Autodesk Fusion 360 part; units mm, degrees
sketch "Sketch1" plane through (0, 0, 0) normal (0, 0, 1) x (1, 0, 0)
  line L0 (0, 0) -> (74, 0)
  line L1 (74, 0) -> (74, 83)
  line L2 (74, 83) -> (0, 83)
  line L3 (0, 83) -> (0, 0)
  dimension "d6" = 74
  dimension "d7" = 83
extrude "Extrude1" add sketch "Sketch1" along normal blind 5
sketch "Sketch2" plane through (0, 0, 0) normal (0, -1, 0) x (1, 0, 0)
  line L0 (0, 0) -> (74, 0)
  line L1 (74, 0) -> (74, 5)
  line L2 (74, 5) -> (0, 5)
  line L3 (0, 5) -> (0, 0)
  line L4 (0, 5) -> (6.7273, 5)
  line L5 (6.7273, 5) -> (6.7273, 0)
  line L6 (6.7273, 0) -> (0, 0)
  line L7 (0, 0) -> (0, 5)
  line L8 (20.1818, 0) -> (13.4545, 0)
  line L9 (13.4545, 0) -> (13.4545, 5)
  line L10 (20.1818, 5) -> (20.1818, 0)
  line L11 (13.4545, 5) -> (20.1818, 5)
  line L12 (33.6364, 0) -> (26.9091, 0)
  line L13 (26.9091, 0) -> (26.9091, 5)
  line L14 (33.6364, 5) -> (33.6364, 0)
  line L15 (26.9091, 5) -> (33.6364, 5)
  line L16 (47.0909, 0) -> (40.3636, 0)
  line L17 (40.3636, 0) -> (40.3636, 5)
  line L18 (47.0909, 5) -> (47.0909, 0)
  line L19 (40.3636, 5) -> (47.0909, 5)
  line L20 (60.5455, 0) -> (53.8182, 0)
  line L21 (53.8182, 0) -> (53.8182, 5)
  line L22 (60.5455, 5) -> (60.5455, 0)
  line L23 (53.8182, 5) -> (60.5455, 5)
  line L24 (74, 0) -> (67.2727, 0)
  line L25 (67.2727, 0) -> (67.2727, 5)
  line L26 (74, 5) -> (74, 0)
  line L27 (67.2727, 5) -> (74, 5)
  dimension "d10" = 6.7273
  dimension "d13" = 67.2727
  dimension "d14" = 0
extrude "Extrude2" add sketch "Sketch2" along normal blind 5 contours L0 L2 L3 L4 L5 L6 L7 | L0 L2 L8 L9 L10 L11 | L0 L2 L12 L13 L14 L15 | L0 L2 L16 L17 L18 L19 | L0 L2 L20 L21 L22 L23 | L0 L1 L2 L24 L25 L26 L27
sketch "Sketch3" plane through (0, 83, 0) normal (0, 1, 0) x (-1, 0, 0)
  line L0 (-74, 0) -> (0, 0)
  line L1 (0, 0) -> (0, 5)
  line L2 (0, 5) -> (-74, 5)
  line L3 (-74, 5) -> (-74, 0)
  line L4 (-74, 5) -> (-67.2727, 5)
  line L5 (-67.2727, 5) -> (-67.2727, 0)
  line L6 (-67.2727, 0) -> (-74, 0)
  line L7 (-74, 0) -> (-74, 5)
  line L8 (-53.8182, 0) -> (-60.5455, 0)
  line L9 (-60.5455, 0) -> (-60.5455, 5)
  line L10 (-53.8182, 5) -> (-53.8182, 0)
  line L11 (-60.5455, 5) -> (-53.8182, 5)
  line L12 (-40.3636, 0) -> (-47.0909, 0)
  line L13 (-47.0909, 0) -> (-47.0909, 5)
  line L14 (-40.3636, 5) -> (-40.3636, 0)
  line L15 (-47.0909, 5) -> (-40.3636, 5)
  line L16 (-26.9091, 0) -> (-33.6364, 0)
  line L17 (-33.6364, 0) -> (-33.6364, 5)
  line L18 (-26.9091, 5) -> (-26.9091, 0)
  line L19 (-33.6364, 5) -> (-26.9091, 5)
  line L20 (-13.4545, 0) -> (-20.1818, 0)
  line L21 (-20.1818, 0) -> (-20.1818, 5)
  line L22 (-13.4545, 5) -> (-13.4545, 0)
  line L23 (-20.1818, 5) -> (-13.4545, 5)
  line L24 (0, 0) -> (-6.7273, 0)
  line L25 (-6.7273, 0) -> (-6.7273, 5)
  line L26 (0, 5) -> (0, 0)
  line L27 (-6.7273, 5) -> (0, 5)
  dimension "d17" = 6.7273
  dimension "d20" = 67.2727
  dimension "d21" = 0
extrude "Extrude3" add sketch "Sketch3" along normal blind 5 contours L0 L2 L3 L4 L5 L6 L7 | L0 L2 L8 L9 L10 L11 | L0 L2 L12 L13 L14 L15 | L0 L2 L16 L17 L18 L19 | L0 L2 L20 L21 L22 L23 | L0 L1 L2 L24 L25 L26 L27
sketch "Sketch4" plane through (0, 0, 0) normal (1, 0, 0) x (0, 1, 0)
  line L0 (0, 0) -> (7.5455, 0)
  line L1 (7.5455, 0) -> (7.5455, 5)
  line L2 (7.5455, 5) -> (0, 5)
  line L3 (0, 5) -> (0, 0)
  line L4 (88, 5) -> (-5, 5)
  line L5 (15.0909, 0) -> (22.6364, 0)
  line L6 (22.6364, 0) -> (22.6364, 5)
  line L7 (22.6364, 5) -> (15.0909, 5)
  line L8 (15.0909, 5) -> (15.0909, 0)
  line L9 (30.1818, 0) -> (37.7273, 0)
  line L10 (37.7273, 0) -> (37.7273, 5)
  line L11 (37.7273, 5) -> (30.1818, 5)
  line L12 (30.1818, 5) -> (30.1818, 0)
  line L13 (45.2727, 0) -> (52.8182, 0)
  line L14 (52.8182, 0) -> (52.8182, 5)
  line L15 (52.8182, 5) -> (45.2727, 5)
  line L16 (45.2727, 5) -> (45.2727, 0)
  line L17 (60.3636, 0) -> (67.9091, 0)
  line L18 (67.9091, 0) -> (67.9091, 5)
  line L19 (67.9091, 5) -> (60.3636, 5)
  line L20 (60.3636, 5) -> (60.3636, 0)
  line L21 (75.4545, 0) -> (83, 0)
  line L22 (83, 0) -> (83, 5)
  line L23 (83, 5) -> (75.4545, 5)
  line L24 (75.4545, 5) -> (75.4545, 0)
  dimension "d24" = 7.5455
  dimension "d27" = 75.4545
  dimension "d28" = 0
extrude "Extrude4" add sketch "Sketch4" against normal blind 5
sketch "Sketch5" plane through (74, 0, 0) normal (1, 0, 0) x (0, 1, 0)
  line L0 (-5, 0) -> (88, 0)
  line L1 (88, 0) -> (88, 5)
  line L2 (88, 5) -> (-5, 5)
  line L3 (-5, 5) -> (-5, 0)
  line L4 (0, 0) -> (7.5455, 0)
  line L5 (7.5455, 0) -> (7.5455, 5)
  line L6 (7.5455, 5) -> (0, 5)
  line L7 (0, 5) -> (0, 0)
  line L8 (15.0909, 0) -> (22.6364, 0)
  line L9 (22.6364, 0) -> (22.6364, 5)
  line L10 (22.6364, 5) -> (15.0909, 5)
  line L11 (15.0909, 5) -> (15.0909, 0)
  line L12 (30.1818, 0) -> (37.7273, 0)
  line L13 (37.7273, 0) -> (37.7273, 5)
  line L14 (37.7273, 5) -> (30.1818, 5)
  line L15 (30.1818, 5) -> (30.1818, 0)
  line L16 (45.2727, 0) -> (52.8182, 0)
  line L17 (52.8182, 0) -> (52.8182, 5)
  line L18 (52.8182, 5) -> (45.2727, 5)
  line L19 (45.2727, 5) -> (45.2727, 0)
  line L20 (60.3636, 0) -> (67.9091, 0)
  line L21 (67.9091, 0) -> (67.9091, 5)
  line L22 (67.9091, 5) -> (60.3636, 5)
  line L23 (60.3636, 5) -> (60.3636, 0)
  line L24 (75.4545, 0) -> (83, 0)
  line L25 (83, 0) -> (83, 5)
  line L26 (83, 5) -> (75.4545, 5)
  line L27 (75.4545, 5) -> (75.4545, 0)
  dimension "d31" = 7.5455
  dimension "d34" = 75.4545
  dimension "d35" = 0
extrude "Extrude5" add sketch "Sketch5" along normal blind 5 contours L0 L2 L4 L5 L6 L7 | L0 L2 L8 L9 L10 L11 | L0 L2 L12 L13 L14 L15 | L0 L2 L16 L17 L18 L19 | L0 L2 L20 L21 L22 L23 | L0 L2 L24 L25 L26 L27
extrude "Extrude6" add 1 faces at (38.1212, 25.1515, 5) along direction (0, 0, 1) blind 0.5
sketch "Sketch6" plane through (79, 0, 0) normal (1, 0, 0) x (0, 1, 0)
  line L0 (75.4545, 5.5) -> (75.4545, 0)
  line L1 (75.4545, 0) -> (83, 0)
  line L2 (83, 0) -> (83, 5.5)
  line L3 (83, 5.5) -> (75.4545, 5.5)
sketch "Sketch7" plane through (0, 0, 0) normal (0, 0, 1) x (1, 0, 0)
  line L0 (79, 75.4545) -> (79, 83) construction
  line L1 (79, 83) -> (91, 83) construction
  line L2 (91, 83) -> (101, 83)
  line L3 (101, 83) -> (101, -6)
  line L4 (101, -6) -> (91, -6)
  line L5 (91, -6) -> (91, 83)
  line L6 (91, 83) -> (101, 83)
  line L7 (101, 83) -> (101, 89)
  line L8 (101, 89) -> (91, 89)
  line L9 (91, 89) -> (91, 83)
  line L10 (91, 83) -> (85, 83)
  line L11 (85, 83) -> (85, 89)
  line L12 (85, 89) -> (91, 89)
  line L13 (91, 89) -> (91, 83)
  line L14 (91, -6) -> (85, -6)
  line L15 (85, -6) -> (85, 0)
  line L16 (85, 0) -> (91, 0)
  line L17 (91, 0) -> (91, -6)
  point P0 (79, 83)
  dimension "d40" = 12
  dimension "d41" = 89
  dimension "d42" = 10
  dimension "d43" = 6
  dimension "d44" = 6
  dimension "d45" = 6
  dimension "d46" = 6
  dimension "d47" = 6
sketch "Sketch8" plane through (91, 0, 0) normal (-1, 0, 0) x (0, -1, 0)
  line L0 (-82, 0) -> (0, 0)
  line L1 (0, 0) -> (0, 6.5)
  line L2 (0, 6.5) -> (-82, 6.5)
  line L3 (-82, 6.5) -> (-82, 0)
  line L4 (-74.4545, 6.5) -> (-66.9091, 6.5)
  line L5 (-66.9091, 6.5) -> (-66.9091, 0)
  line L6 (-66.9091, 0) -> (-74.4545, 0)
  line L7 (-74.4545, 0) -> (-74.4545, 6.5)
  line L8 (-51.8182, 0) -> (-59.3636, 0)
  line L9 (-59.3636, 0) -> (-59.3636, 6.5)
  line L10 (-51.8182, 6.5) -> (-51.8182, 0)
  line L11 (-59.3636, 6.5) -> (-51.8182, 6.5)
  line L12 (-36.7273, 0) -> (-44.2727, 0)
  line L13 (-44.2727, 0) -> (-44.2727, 6.5)
  line L14 (-36.7273, 6.5) -> (-36.7273, 0)
  line L15 (-44.2727, 6.5) -> (-36.7273, 6.5)
  line L16 (-21.6364, 0) -> (-29.1818, 0)
  line L17 (-29.1818, 0) -> (-29.1818, 6.5)
  line L18 (-21.6364, 6.5) -> (-21.6364, 0)
  line L19 (-29.1818, 6.5) -> (-21.6364, 6.5)
  line L20 (-6.5455, 0) -> (-14.0909, 0)
  line L21 (-14.0909, 0) -> (-14.0909, 6.5)
  line L22 (-6.5455, 6.5) -> (-6.5455, 0)
  line L23 (-14.0909, 6.5) -> (-6.5455, 6.5)
  dimension "d50" = 7.5455
  dimension "d51" = 7.5455
  dimension "d54" = 60.3636
  dimension "d55" = 0
sketch "Sketch9" plane through (0, 0, 0) normal (0, 0, 1) x (1, 0, 0)
equation "paksus = 5 mm"
equation "laius = 74 mm"
equation "pikkus = 83 mm"
equation "laius_tapp = laius / 11"
equation "pikkus_tapp = pikkus / 11"
equation "d6 = laius"
equation "d7 = pikkus"
equation "d8 = paksus"
equation "d10 = laius_tapp"
equation "d13 = laius - laius_tapp"
equation "d15 = paksus"
equation "d17 = laius_tapp"
equation "d20 = laius - laius_tapp"
equation "d22 = paksus"
equation "d24 = pikkus_tapp"
equation "d27 = pikkus - pikkus_tapp"
equation "d31 = pikkus_tapp"
equation "d34 = pikkus - pikkus_tapp"
equation "d36 = paksus"
equation "d41 = pikkus + 6 mm"
equation "d50 = pikkus_tapp"
equation "d51 = pikkus_tapp"
equation "d54 = pikkus - pikkus_tapp * 3"
Verification items for the finished model (mm, model axes). A direction names the side the tool comes from. Give positions to 0.01 mm unless a question says otherwise; leave off trailing zeros. Loops run counter-clockwise (first coordinate to the right, second up) from the corner with the lowest first, then second, coordinate; pieces in that order, holes last.
1) Sectioned sample at A-A, the plane x = 64. Enter the section's corners in (y, z).
2) Sectioned sample at B-B, the plane y = 72. Enter the section's corners in (x, z).
3) Set-up check for faces 1 (the flat face through (26.909, 85, 3)), 2 (the flat face through (10, 0, 3)), 3 (the flat face through (-2, 7.546, 3)), 4 (the flat face through (76, 83, 3)): record each of +Z, -Z, +X, -X, +Y, -Y from which the full face is reachable in a straight line by a thin tool's end or side.
4) Draft check along X on faces 5 (the flat face through (76, 75.454, 3)), 6 (the flat face through (24, 83, 3)), 7 (the flat face through (37, 0, 3)), 8 (the flat face through (74, 57, 3)). Enter one of: pulls with the +X half, pulls with the -X half, needs draft (parallel to the pull), parting line crosses it, or undercut.
5) Thickness scan on line 1 along Y through (x, z) = (11, 3.75); line 2 along X through (y, z) = (13.5, 3.5). Record the ranges inside material, lowest first.
6) Depth check by flat-ended pin: pin 1 Ø2.5 at (y, z) = (-1.5, 1.5) entering from +X; pin 2 Ø1.6 at (y, z) = (13, 3) entering from -X; pin 3 Ø1.5 at (x, z) = (76.5, 3.5) entering from -Y. Enter the tip coordinate at first touch or a pass-through.
Answers:
1. outline: (0, 0) - (83, 0) - (83, 5.5) - (0, 5.5) - close
2. outline: (0, 0) - (74, 0) - (74, 5.5) - (0, 5.5) - close
3. face 1: +Z, -Z, +Y
3. face 2: +Z, -Z, -Y
3. face 3: +Z, -Z, -X
3. face 4: +Z, -Z, +X, +Y
4. face 5: needs draft
4. face 6: undercut
4. face 7: undercut
4. face 8: pulls with the +X half
5. line 1: y = 0 to 83
5. line 2: x = 0 to 74
6. pin 1: stops at x = 74
6. pin 2: stops at x = 0
6. pin 3: stops at y = 0
